Source: CAD feature listing. Evaluate the final solid. Frame: model axes, mm. A direction names the side the tool comes from. Give positions to 0.01 mm unless a question says otherwise; leave off trailing zeros. Write each loop counter-clockwise with the first axis right and the second up, starting at its lowest first coordinate (ties: lowest second). Pieces come first, ordered by that corner, then holes. Notation, with made-up numbers: (74, 62) - (97, 62) arc R23 ccw to (97, 82) - close; hole circle Ø6 at (-11.5, -19). An arc over 180 degrees is marked (long way). One line per question, with ' | ' between items. Start each with the question number.
(1) Section B-B, the plane x = 1. Return loops of the section in (y, z).
(2) Ray query, line 1 (X direction, y = 163, z = 9.15); line 2 (Y direction, x = -32.5, z = 9.45); line 3 (X direction, y = 92.5, z = 1.75). Return the intervals inside material, ascending. Write a range as [from, to].
(3) Access query for faces 1 (the flat face through (29.7, 43.1, 7)), 2 (the cylindrical face through (-20.23, 201.89, 4.62)), 3 (the flat face through (0, 192, 5)). Directions: +Z, -Z, +X, -X, +Y, -Y. A direction counts if a zero-diameter tool reaches every point of the face in a straight line with its end or side. Return the directions, or none.
(4) Section C-C, the plane y = 163. Return loops of the section in (x, z).
(5) Draft query along X for faces 4 (the flat face through (-37.5, 106, 6)), 5 (the cylindrical face through (-15.273, 204.582, 5.81)), 6 (the flat face through (-18, 124, 0)), 7 (the cylindrical face through (33.053, 167.214, 4.212)). Return one class per face: +X half, -X half, draft (parallel to the pull), parting line (faces both ways), or undercut.
(6) Section A-A, the plane y = 73. Return loops of the section in (x, z).
(7) Pin query (flat end, axial travel): pin 1 (6 mm diameter, centred on x = -11, z = 3.5, fed in from -Y); pin 2 (7 mm diameter, centred on x = -34.5, y = 164.5, fed in from -Z); pin 3 (2 mm diameter, centred on y = 148, z = 5.8, fed in from +X); pin 4 (1.5 mm diameter, centred on y = 88, z = 5.8, fed in from +X). Return the tip coordinate at first contact, or that it passes through.
```python
from build123d import *

# Parameters (mm, degrees)
BOSS_EXTRUDE1_DEPTH                                 = 10
M5_TAPPED_HOLE1_D                                   = 4.1
M5_TAPPED_HOLE1_DEPTH                               = 14
M5_TAPPED_HOLE1_TIP                                 = 1.231764269
CUT_EXTRUDE1_REACH                                  = 12
SKETCH4_W                                           = 35
SKETCH4_H                                           = 130
FILLET1_R                                           = 2
SKETCH6_W                                           = 15
SKETCH6_H                                           = 210
CUT_EXTRUDE2_DEPTH                                  = 1.5
SKETCH7_W                                           = 45
SKETCH7_H                                           = 15
CUT_EXTRUDE3_DEPTH                                  = 1.5
CBORE_FOR_M5_HEX_SOCKET_HEAD_CAP_SCREW1_D           = 5.2
CBORE_FOR_M5_HEX_SOCKET_HEAD_CAP_SCREW1_CBORE_D     = 8.5
CBORE_FOR_M5_HEX_SOCKET_HEAD_CAP_SCREW1_CBORE_DEPTH = 5.5
M5_TAPPED_HOLE2_D                                   = 4.2
M5_TAPPED_HOLE2_DEPTH                               = 16
M5_TAPPED_HOLE2_TIP                                 = 1.2618073
M5_TAPPED_HOLE3_D                                   = 4.2
M5_TAPPED_HOLE3_DEPTH                               = 103.56
M5_TAPPED_HOLE3_TIP                                 = 1.2618073
SKETCH14_W                                          = 45
SKETCH14_H                                          = 18
CUT_EXTRUDE4_DEPTH                                  = 5
FILLET2_R                                           = 2
SKETCH15_W                                          = 15
SKETCH15_H                                          = 18
CUT_EXTRUDE6_DEPTH                                  = 5
TAP_DRILL_FOR_M5_TAP1_D                             = 5.2
TAP_DRILL_FOR_M5_TAP1_DEPTH                         = 46
TAP_DRILL_FOR_M5_TAP1_CSINK_D                       = 6
TAP_DRILL_FOR_M5_TAP1_CSINK_ANGLE                   = 90
TAP_DRILL_FOR_M5_TAP1_TIP                           = 1.562237609
CHAMFER1_SIZE                                       = 1
M3_TAPPED_HOLE1_AT_2_COUNT                          = 2
M3_TAPPED_HOLE1_AT_2_PITCH                          = 50
M3_TAPPED_HOLE1_AT_3_COUNT                          = 2
M3_TAPPED_HOLE1_AT_3_PITCH                          = 80
M3_TAPPED_HOLE1_AT_4_COUNT                          = 2
M3_TAPPED_HOLE1_AT_4_PITCH                          = 110
M3_TAPPED_HOLE1_AT_5_COUNT                          = 2
M3_TAPPED_HOLE1_AT_5_PITCH                          = 170
M3_TAPPED_HOLE2_D                                   = 2.5


with BuildPart() as part:
    # Sketch1 → Boss-Extrude1 (new body)
    with BuildSketch(Plane.XY):
        Polygon((-37.5, 0), (0, 0), (37.5, 0), (37.5, 210), (0, 210), (-37.5, 210), align=None)
    extrude(amount=BOSS_EXTRUDE1_DEPTH)

    # M5 Tapped Hole1
    with Locations(Plane(origin=(30, 193, 0), x_dir=(-1, 0, 0), z_dir=(0, 0, -1))):
        with Locations((0, 0), (0, -60), (0, -120), (0, -180), (60, -180), (60, -120), (60, -60), (60, 0)):
            Hole(M5_TAPPED_HOLE1_D / 2, depth=M5_TAPPED_HOLE1_DEPTH)
            with Locations((0, 0, -(M5_TAPPED_HOLE1_DEPTH + M5_TAPPED_HOLE1_TIP / 2))):  # 118° drill point
                Cone(0, M5_TAPPED_HOLE1_D / 2, M5_TAPPED_HOLE1_TIP, mode=Mode.SUBTRACT)

    # Sketch4 → Cut-Extrude1 (cut, up to next)
    with BuildSketch(Plane(origin=(0, 0, 0), x_dir=(-1, 0, 0), z_dir=(0, 0, -1)), mode=Mode.PRIVATE) as cut_extrude1_sk1:
        with Locations((0, 127)):
            Rectangle(SKETCH4_W, SKETCH4_H)
    cut_extrude1_tool1 = extrude(cut_extrude1_sk1.sketch, amount=-CUT_EXTRUDE1_REACH, mode=Mode.PRIVATE) & part.part
    add(cut_extrude1_tool1.solids().sort_by_distance((0, 127, 0))[0], mode=Mode.SUBTRACT)

    # Fillet1
    fillet1_edges = [part.edges().sort_by_distance(p)[0] for p in [
        (17.5, 62, 5),
        (17.5, 192, 5),
        (-17.5, 192, 5),
        (-17.5, 62, 5),
    ]]
    fillet(fillet1_edges, radius=FILLET1_R)

    # Sketch6 → Cut-Extrude2 (cut)
    with BuildSketch(Plane(origin=(0, 0, 0), x_dir=(-1, 0, 0), z_dir=(0, 0, -1))):
        with Locations((-30, 105)):
            Rectangle(SKETCH6_W, SKETCH6_H)
        with Locations((30, 105)):
            Rectangle(SKETCH6_W, SKETCH6_H)
    extrude(amount=-CUT_EXTRUDE2_DEPTH, mode=Mode.SUBTRACT)

    # Sketch7 → Cut-Extrude3 (cut)
    with BuildSketch(Plane(origin=(0, 0, 0), x_dir=(-1, 0, 0), z_dir=(0, 0, -1))):
        with Locations((0, 202.5)):
            Rectangle(SKETCH7_W, SKETCH7_H)
    extrude(amount=-CUT_EXTRUDE3_DEPTH, mode=Mode.SUBTRACT)

    # CBORE for M5 Hex Socket Head Cap Screw1 (through all)
    with Locations(Plane(origin=(32.5, 205, 1.5), x_dir=(-1, 0, 0), z_dir=(0, 0, -1))):
        with Locations((0, 0), (0, -42), (0, -102), (0, -162), (0, -200), (65, -200), (65, -162), (65, -102), (65, -42), (65, 0)):
            CounterBoreHole(CBORE_FOR_M5_HEX_SOCKET_HEAD_CAP_SCREW1_D / 2, CBORE_FOR_M5_HEX_SOCKET_HEAD_CAP_SCREW1_CBORE_D / 2, CBORE_FOR_M5_HEX_SOCKET_HEAD_CAP_SCREW1_CBORE_DEPTH)

    # M5 Tapped Hole2
    with Locations(Plane(origin=(-22, 210, 5.75), x_dir=(0, 0, 1), z_dir=(0, 1, 0))):
        with Locations((0, 0), (0, 44)):
            Hole(M5_TAPPED_HOLE2_D / 2, depth=M5_TAPPED_HOLE2_DEPTH)
            with Locations((0, 0, -(M5_TAPPED_HOLE2_DEPTH + M5_TAPPED_HOLE2_TIP / 2))):  # 118° drill point
                Cone(0, M5_TAPPED_HOLE2_D / 2, M5_TAPPED_HOLE2_TIP, mode=Mode.SUBTRACT)

    # M5 Tapped Hole3
    with Locations(Plane(origin=(15, 202.5, 1.5), x_dir=(-1, 0, 0), z_dir=(0, 0, -1))):
        with Locations((0, 0), (30, 0)):
            Hole(M5_TAPPED_HOLE3_D / 2, depth=M5_TAPPED_HOLE3_DEPTH)
            with Locations((0, 0, -(M5_TAPPED_HOLE3_DEPTH + M5_TAPPED_HOLE3_TIP / 2))):  # 118° drill point
                Cone(0, M5_TAPPED_HOLE3_D / 2, M5_TAPPED_HOLE3_TIP, mode=Mode.SUBTRACT)

    # Sketch14 → Cut-Extrude4 (cut)
    with BuildSketch(Plane(origin=(0, 0, 0), x_dir=(-1, 0, 0), z_dir=(0, 0, -1))):
        with Locations((0, 44)):
            Rectangle(SKETCH14_W, SKETCH14_H)
    extrude(amount=-CUT_EXTRUDE4_DEPTH, mode=Mode.SUBTRACT)

    # Fillet2
    fillet2_edges = [part.edges().sort_by_distance(p)[0] for p in [
        (22.5, 35, 3.25),
        (22.5, 53, 3.25),
        (-22.5, 53, 3.25),
        (-22.5, 35, 3.25),
    ]]
    fillet(fillet2_edges, radius=FILLET2_R)

    # Sketch15 → Cut-Extrude6 (cut)
    with BuildSketch(Plane(origin=(0, 0, 0), x_dir=(-1, 0, 0), z_dir=(0, 0, -1))):
        with Locations((0, 62)):
            Rectangle(SKETCH15_W, SKETCH15_H)
    extrude(amount=-CUT_EXTRUDE6_DEPTH, mode=Mode.SUBTRACT)

    # Tap Drill for M5 Tap1
    with Locations(Plane(origin=(16, 42.5, 5), x_dir=(-1, 0, 0), z_dir=(0, 0, -1))):
        with Locations((0, 0), (32, 0)):
            CounterSinkHole(TAP_DRILL_FOR_M5_TAP1_D / 2, TAP_DRILL_FOR_M5_TAP1_CSINK_D / 2, depth=TAP_DRILL_FOR_M5_TAP1_DEPTH, counter_sink_angle=TAP_DRILL_FOR_M5_TAP1_CSINK_ANGLE)
            with Locations((0, 0, -(TAP_DRILL_FOR_M5_TAP1_DEPTH + TAP_DRILL_FOR_M5_TAP1_TIP / 2))):  # 118° drill point
                Cone(0, TAP_DRILL_FOR_M5_TAP1_D / 2, TAP_DRILL_FOR_M5_TAP1_TIP, mode=Mode.SUBTRACT)

    # Chamfer1
    chamfer1_edges = [part.edges().sort_by_distance(p)[0] for p in [
        (-22.5, 195, 0.75),
        (22.5, 195, 0.75),
        (-22.5, 35, 0.75),
        (-22.5, 53, 0.75),
        (22.5, 35, 0.75),
        (22.5, 53, 0.75),
        (7.5, 62, 2.5),
        (7.5, 53, 2.5),
        (-7.5, 62, 2.5),
        (-7.5, 53, 2.5),
    ]]
    chamfer(chamfer1_edges, length=CHAMFER1_SIZE)

    # Sketch20 → M3 Tapped Hole1 (revolve, cut)
    with BuildSketch(Plane(origin=(-37.5, 198, 5.8), x_dir=(0, 0, 1), z_dir=(0, 1, 0))):
        Polygon((0, 0), (0, 9.251075774), (1.25, 8.5), (1.25, 0), align=None)
    m3_tapped_hole1 = revolve(axis=Axis((-43.85, 198, 5.8), (1, 0, 0)), mode=Mode.SUBTRACT)

    # M3 Tapped Hole1 at 2: M3 Tapped Hole1 ×2
    with Locations(*[(0, -i * M3_TAPPED_HOLE1_AT_2_PITCH, 0) for i in range(1, M3_TAPPED_HOLE1_AT_2_COUNT)]):
        add(m3_tapped_hole1, mode=Mode.SUBTRACT)

    # M3 Tapped Hole1 at 3: M3 Tapped Hole1 ×2
    with Locations(*[(0, -i * M3_TAPPED_HOLE1_AT_3_PITCH, 0) for i in range(1, M3_TAPPED_HOLE1_AT_3_COUNT)]):
        add(m3_tapped_hole1, mode=Mode.SUBTRACT)

    # M3 Tapped Hole1 at 4: M3 Tapped Hole1 ×2
    with Locations(*[(0, -i * M3_TAPPED_HOLE1_AT_4_PITCH, 0) for i in range(1, M3_TAPPED_HOLE1_AT_4_COUNT)]):
        add(m3_tapped_hole1, mode=Mode.SUBTRACT)

    # M3 Tapped Hole1 at 5: M3 Tapped Hole1 ×2
    with Locations(*[(0, -i * M3_TAPPED_HOLE1_AT_5_PITCH, 0) for i in range(1, M3_TAPPED_HOLE1_AT_5_COUNT)]):
        add(m3_tapped_hole1, mode=Mode.SUBTRACT)

    # Mirror1: M3 Tapped Hole1 across plane
    add(m3_tapped_hole1.mirror(Plane(origin=(0, 0, 0), x_dir=(0, 0, 1), z_dir=(1, 0, 0))), mode=Mode.SUBTRACT)

    # Mirror1 copy 1 sketch → Mirror1 copy 1 (revolve, cut)
    with BuildSketch(Plane(origin=(37.5, 148, 5.8), x_dir=(0, 0, 1), z_dir=(0, 1, 0))):
        Polygon((0, 0), (0, -9.251075774), (1.25, -8.5), (1.25, 0), align=None)
    revolve(axis=Axis((43.85, 148, 5.8), (1, 0, 0)), mode=Mode.SUBTRACT)

    # Mirror1 copy 2 sketch → Mirror1 copy 2 (revolve, cut)
    with BuildSketch(Plane(origin=(37.5, 118, 5.8), x_dir=(0, 0, 1), z_dir=(0, 1, 0))):
        Polygon((0, 0), (0, -9.251075774), (1.25, -8.5), (1.25, 0), align=None)
    revolve(axis=Axis((43.85, 118, 5.8), (1, 0, 0)), mode=Mode.SUBTRACT)

    # Mirror1 copy 3 sketch → Mirror1 copy 3 (revolve, cut)
    with BuildSketch(Plane(origin=(37.5, 88, 5.8), x_dir=(0, 0, 1), z_dir=(0, 1, 0))):
        Polygon((0, 0), (0, -9.251075774), (1.25, -8.5), (1.25, 0), align=None)
    revolve(axis=Axis((43.85, 88, 5.8), (1, 0, 0)), mode=Mode.SUBTRACT)

    # Mirror1 copy 4 sketch → Mirror1 copy 4 (revolve, cut)
    with BuildSketch(Plane(origin=(37.5, 28, 5.8), x_dir=(0, 0, 1), z_dir=(0, 1, 0))):
        Polygon((0, 0), (0, -9.251075774), (1.25, -8.5), (1.25, 0), align=None)
    revolve(axis=Axis((43.85, 28, 5.8), (1, 0, 0)), mode=Mode.SUBTRACT)

    # M3 Tapped Hole2 (through all)
    with Locations(Plane(origin=(7.5, 5, 0), x_dir=(-1, 0, 0), z_dir=(0, 0, -1))):
        with Locations((0, 0), (10, 0)):
            Hole(M3_TAPPED_HOLE2_D / 2)


solid = part.part
```
Check sheet entries:
1) outline: (0, 0) - (35, 0) - (35, 5) - (62, 5) - (62, 10) - (0, 10) - close; (192, 0) - (195, 0) - (195, 1.5) - (210, 1.5) - (210, 10) - (192, 10) - close
2) line 1: [-37.5, -35.1], [-29.9, -17.5], [17.5, 29.9], [35.1, 37.5] | line 2: [0, 2.4], [7.6, 40.4], [45.6, 100.4], [105.6, 160.4], [165.6, 202.4], [207.6, 210] | line 3: [-37.5, -17.5], [17.5, 37.5]
3) face 1: -Z | face 2: +Y | face 3: +Z, -Z
4) outline: (-37.5, 1.5) - (-36.75, 1.5) - (-36.75, 7) - (-35.1, 7) - (-35.1, 10) - (-37.5, 10) - close; (-29.9, 7) - (-28.25, 7) - (-28.25, 1.5) - (-22.5, 1.5) - (-22.5, 0) - (-17.5, 0) - (-17.5, 10) - (-29.9, 10) - close; (17.5, 0) - (22.5, 0) - (22.5, 1.5) - (28.25, 1.5) - (28.25, 7) - (29.9, 7) - (29.9, 10) - (17.5, 10) - close; (35.1, 7) - (36.75, 7) - (36.75, 1.5) - (37.5, 1.5) - (37.5, 10) - (35.1, 10) - close
5) face 4: -X half | face 5: undercut | face 6: draft | face 7: undercut
6) outline: (-37.5, 1.5) - (-32.05, 1.5) - (-32.05, 10) - (-37.5, 10) - close; (-27.95, 1.5) - (-22.5, 1.5) - (-22.5, 0) - (-17.5, 0) - (-17.5, 10) - (-27.95, 10) - close; (17.5, 0) - (22.5, 0) - (22.5, 1.5) - (27.95, 1.5) - (27.95, 10) - (17.5, 10) - close; (32.05, 1.5) - (37.5, 1.5) - (37.5, 10) - (32.05, 10) - close
7) pin 1: y = 0 | pin 2: z = 1.5 | pin 3: x = 28.85 | pin 4: x = 28.7
